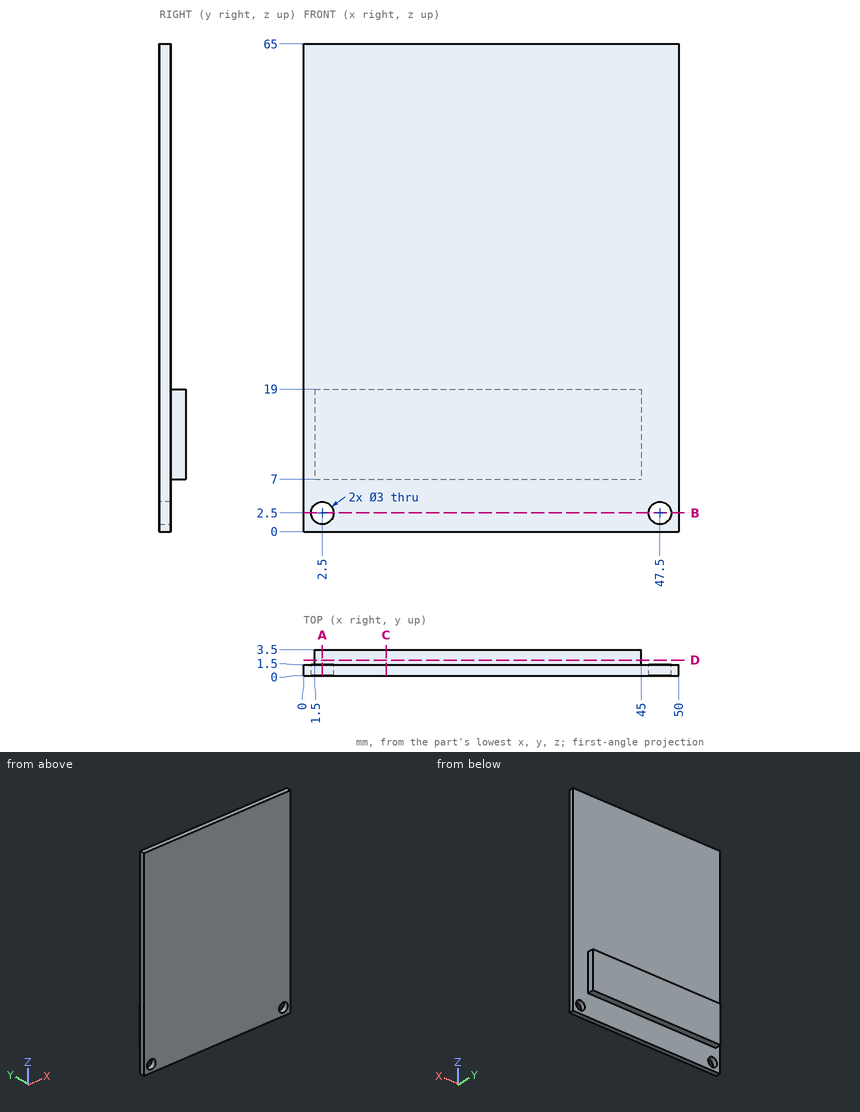
Verification items for this drawing (mm, ordinates from the low corner). Coordinates: 2 decimals unless noted, no trailing zeros. Loops run counter-clockwise (first coordinate to the right, second up) from the corner with the lowest first, then second, coordinate; pieces in that order, holes last.
Item 1: Sectioned sample at A-A, the plane x = 2.5. Record the boundary of the cut face in (y, z).
Item 2: Go/stop test with flat-tipped pins: pin 1 Ø2.5 at (x, z) = (2.5, 2.5) entering from -Y; pin 2 Ø1 at (y, z) = (2.5, 10) entering from +X; pin 3 Ø1.5 at (x, z) = (17, 23.5) entering from +Y; pin 4 Ø1.6 at (y, z) = (2.5, 14) entering from -X. Record where each tip stops, or that it passes through.
Item 3: Sectioned sample at C-C, the plane x = 11. Record the boundary of the cut face in (y, z), then the cut area to 4 significant figures.
Item 4: Thickness scan on line 1 (X direction, y = 0.85, z = 2.5); line 2 (Y direction, x = 13, z = 19.5); line 3 (X direction, y = 1.7, z = 13.5). Record the ranges inside material, lowest first.
Item 5: Sectioned sample at D-D, the plane y = 2.1. Record the boundary of the cut face in (x, z).
Item 6: Sectioned sample at B-B, the plane z = 2.5. Record the boundary of the cut face in (x, y).
Check result:
1. outline: (0, 0) - (1.5, 0) - (1.5, 1) - (0, 1) - close; (0, 4) - (1.5, 4) - (1.5, 7) - (3.5, 7) - (3.5, 19) - (1.5, 19) - (1.5, 65) - (0, 65) - close
2. pin 1: passes through
2. pin 2: stops at x = 45
2. pin 3: stops at y = 1.5
2. pin 4: stops at x = 1.5
3. outline: (0, 0) - (1.5, 0) - (1.5, 7) - (3.5, 7) - (3.5, 19) - (1.5, 19) - (1.5, 65) - (0, 65) - close
3. area: 121.5 mm2
4. line 1: x = 0 to 1, 4 to 46, 49 to 50
4. line 2: y = 0 to 1.5
4. line 3: x = 1.5 to 45
5. outline: (1.5, 7) - (45, 7) - (45, 19) - (1.5, 19) - close
6. outline: (0, 0) - (1, 0) - (1, 1.5) - (0, 1.5) - close; (4, 0) - (46, 0) - (46, 1.5) - (4, 1.5) - close; (49, 0) - (50, 0) - (50, 1.5) - (49, 1.5) - close
